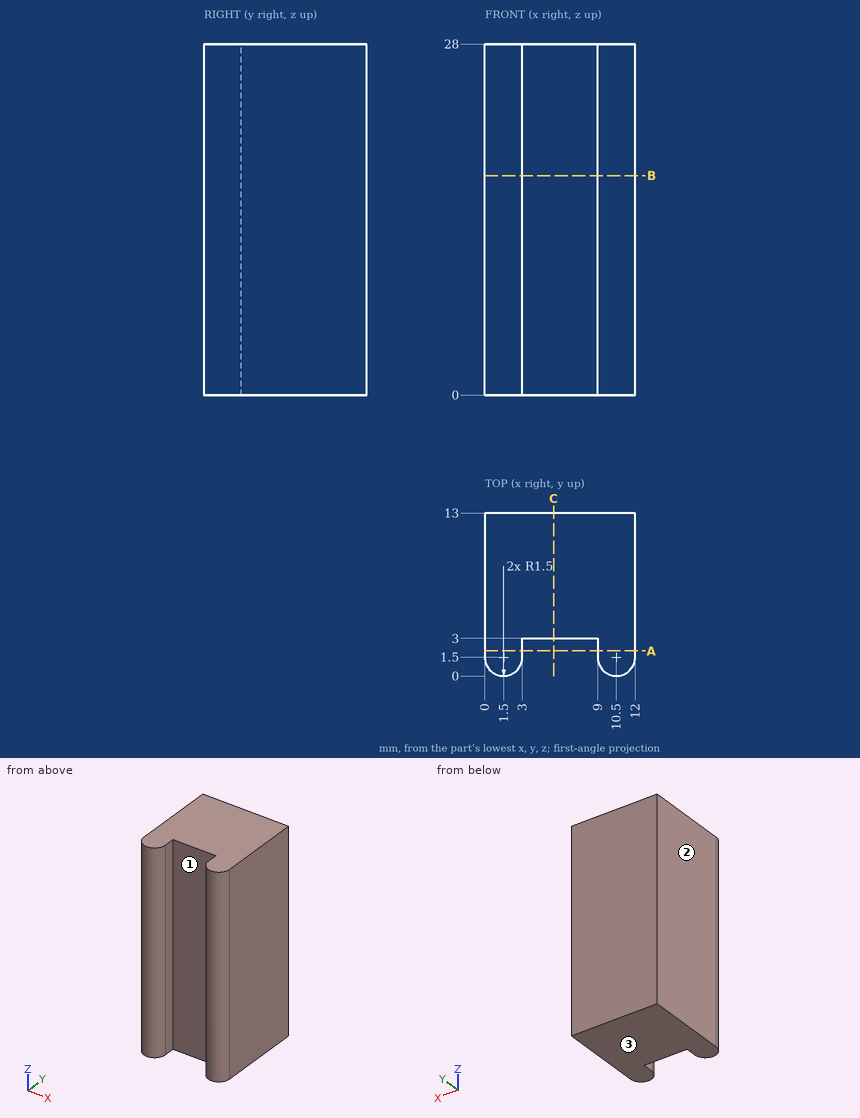
Part print with two shaded views. Sizes in mm from the minimum x, y, z corner. Round coordinates to 2 decimals unless told otherwise and drop trailing zeros. Loops run counter-clockwise (first coordinate to the right, second up) from the corner with the lowest first, then second, coordinate; pieces in that order, holes last. Notation, with made-up numbers: (3.25, -0.5) - (61.25, -0.5) arc R13 ccw to (61.25, 21.5) - close; hole circle Ø10 at (-35.75, -27). An arc over 180 degrees is marked (long way). Put each result on its own line as item: value.
1. Wall check: line 1 (Y direction, x = 4, z = 21); line 2 (Y direction, x = 10, z = 16.5). Give the ranges that are in metal, low to high.
Geometry check:
line 1: 3 to 13
line 2: 0.09 to 13
2. Slice it at C-C on x = 5.5. List the corners of the cut face in (y, z).
Geometry check:
outline: (3, 0) - (13, 0) - (13, 28) - (3, 28) - close
3. Slice it at A-A on y = 2. List the corners of the cut face in (x, z), and give its area (3 significant figures).
Geometry check:
outline: (0, 0) - (3, 0) - (3, 28) - (0, 28) - close; (9, 0) - (12, 0) - (12, 28) - (9, 28) - close
area: 168 mm²
4. Two-plate mould, pull along X, no slides. Class the marked faces 1, 2 and 3: released by +X, released by -X, zero draft, split by the parting line, or undercut.
Geometry check:
face 1: undercut
face 2: released by -X
face 3: zero draft
5. Slice it at B-B on z = 17.5. List the corners of the cut face in (x, y).
Geometry check:
outline: (0, 1.5) arc R1.5 ccw to (3, 1.5) - (3, 3) - (9, 3) - (9, 1.5) arc R1.5 ccw to (12, 1.5) - (12, 13) - (0, 13) - close
6. Pin check, flat tip, straight feed: P1, Ø3, axis at x = 7, z = 16.5, coming from the -Y side. Stop position of the tip, or through.
Geometry check:
P1: y = 3
